Verification items for the finished model (mm, model axes). Face numbers are marked on the shaded views. A direction names the side the tool comes from. Round coordinates to 2 decimals unless told otherwise and drop trailing zeros. Write item = value, one per line.
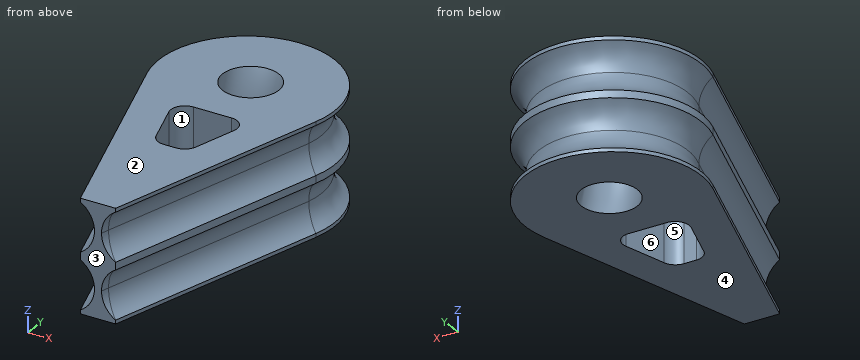
```python
from build123d import *

# Parameters (mm, degrees)
F1_DEPTH  = 4
F8_R      = 4
F11_DEPTH = 16
F12_R     = 2


with BuildPart() as f1:
    # F0 (on Top) → F1 (new body)
    with BuildSketch(Plane.XY):
        with BuildLine():
            Line((2.5, -35), (11.9675303731, -3.6094621162))
            ThreePointArc((11.9675303731, -3.6094621162), (0, 12.5), (-11.9675303731, -3.6094621162))
            Line((-11.9675303731, -3.6094621162), (-2.5, -35))
            Line((-2.5, -35), (2.5, -35))
        make_face()
    extrude(amount=F1_DEPTH)

    # F4: sweep along a path in F4_path
    with BuildLine(Plane(origin=(-11.9675303731, -3.6094621162, 4), x_dir=(0, 1, 0), z_dir=(0, 0, 1))) as f4_path:
        Line((-31.3905378838, -9.4675303731), (0, 0))
        ThreePointArc((0, 0), (16.1094621162, -11.9675303731), (0, -23.9350607463))
        Line((0, -23.9350607463), (-31.3905378838, -14.4675303731))
        Line((-31.3905378838, -14.4675303731), (-38.5466098599, -12.309226204))
    # F3 (on face) → F4 (sweep, cut)
    with BuildSketch(Plane.XZ.offset(35)):
        with BuildLine():
            ThreePointArc((-2.5, 0.5358983849), (-1.0358983849, 2), (-0.5, 4))
            Line((-0.5, 4), (-2.5, 4))
            Line((-2.5, 4), (-2.5, 0.5358983849))
        make_face()
    sweep(path=f4_path.line, mode=Mode.SUBTRACT)

    # F5: F1 across face


with BuildPart() as f1_1:
    add(f1.part)
    add(f1.part.mirror(Plane(origin=(-0.0002119215, -7.1160026753, 4), x_dir=(1, 0, 0), z_dir=(0, 0, 1))))

    # F6: F1 across face


with BuildPart() as f1_2:
    add(f1_1.part)
    add(f1_1.part.mirror(Plane(origin=(0, -7.6972152999, 0), x_dir=(1, 0, 0), z_dir=(0, 0, -1))))

    # F9: sweep along a path in F7
    with BuildLine(Plane.YZ) as f9_path:
        CenterArc((20, 0), 20, 0, 360)
    # F8 (on face) → F9 (sweep, cut)
    with BuildSketch(Plane(origin=(0, 0, -8), x_dir=(1, 0, 0), z_dir=(0, 0, -1))):
        with Locations((0, -0.9167455137)):
            Circle(F8_R)
    sweep(path=f9_path.line, mode=Mode.SUBTRACT)

    # F10 (on face) → F11 (cut, through all)
    with BuildSketch(Plane(origin=(0, 0, -8), x_dir=(1, 0, 0), z_dir=(0, 0, -1))):
        Polygon((5.3957497615, 8.0832544863), (2.3797038408, 18.0832544863), (-2.3797038408, 18.0832544863), (-5.3957497615, 8.0832544863), align=None)
    extrude(amount=-F11_DEPTH, mode=Mode.SUBTRACT)

    # F12
    f12_edges = [f1_2.edges().sort_by_distance(p)[0] for p in [
        (-5.39575, -8.083254, 0),
        (5.39575, -8.083254, 0),
        (-2.379704, -18.083254, 0),
        (2.379704, -18.083254, 0),
    ]]
    fillet(f12_edges, radius=F12_R)


solid = f1_2.part
```
(1) Go/stop test with flat-tipped pins: pin 1 Ø1 at (x, z) = (-1, 6.5) entering from +Y; pin 2 Ø8 at (y, z) = (0.5, -5.5) entering from -X; pin 3 Ø3 at (x, z) = (-3, 4.5) entering from +Y; pin 4 Ø1 at (x, z) = (-5, -4.5) entering from +Y. Record where each tip stops, or that it passes through.
Filled sheet:
pin_1 = 11.84
pin_2 = -12.5
pin_3 = 10.78
pin_4 = 9.64
(2) Sectioned sample at A-A, the plane z = -7. Count the separate pieces of the cut face and the enclosed holes in it, and give its area (3 significant figures).
Filled sheet:
separate_pieces = 1
enclosed_holes = 2
area = 597 mm2
(3) Material ranges on probe 1 along X at (y, z) = (-1.5, 5.25); probe 2 along X at (y, z) = (-1.5, -1.5); probe 3 along X at (y, z) = (8, -1), recorded low to high. Write a range as from..to.
Filled sheet:
probe_1 = -10.68..-3.69, 3.69..10.68
probe_2 = -11.33..-3.89, 3.89..11.33
probe_3 = -8.79..8.79
(4) Draft check along Y on the marked faces 3, 4, 5 and 6. Enter one of: released by +Y, released by -Y, zero draft, split by the parting line, or undercut.
Filled sheet:
face_3 = released by -Y
face_4 = zero draft
face_5 = undercut
face_6 = undercut
(5) Set-up check for the marked faces 1 and 2: record each of +Z, -Z, +X, -X, +Y, -Y from which the full face is reachable in a straight line by a thin tool's end or side.
Filled sheet:
face_1 = +Z, -Z
face_2 = +Z, +X, -X, +Y, -Y
